Check sheet for the modelled part. Datum: model origin and axes. Units: mm. Face numbers are marked on the shaded views. A direction names the side the tool comes from. Round coordinates to 2 decimals unless told otherwise and drop trailing zeros. Write each loop counter-clockwise with the first axis right and the second up, starting at its lowest first coordinate (ties: lowest second). Pieces come first, ordered by that corner, then holes. Notation, with made-up numbers: (11, 66.25) -> (36, 66.25) arc R22 cw to (36, 99.25) -> close; hole circle Ø8 at (73, 68.5). An arc over 180 degrees is marked (long way). One line per item, written item: value. Start each with the question number.
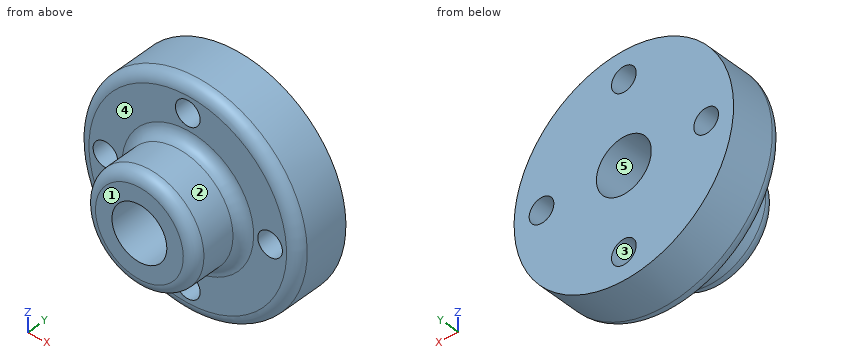
```python
from build123d import *

# Parameters (mm, degrees)
SKETCH1_R           = 254
BOSS_EXTRUDE1_DEPTH = 254
SKETCH2_R           = 508
BOSS_EXTRUDE2_DEPTH = 254
SKETCH3_R           = 127
CUT_EXTRUDE1_DEPTH  = 880.881810245
SKETCH4_R           = 57.15
CUT_EXTRUDE2_DEPTH  = 763
FILLET1_R           = 50.8


with BuildPart() as part:
    # Sketch1 → Boss-Extrude1 (new body)
    with BuildSketch(Plane(origin=(0, 0, 0), x_dir=(1, 0, 0), z_dir=(0, 1, 0))):
        with Locations(Location((0, 0, 0), (0, 0, 270))):
            Circle(SKETCH1_R)
    extrude(amount=BOSS_EXTRUDE1_DEPTH)

    # Sketch2 → Boss-Extrude2 (add)
    with BuildSketch(Plane(origin=(0, 254, 0), x_dir=(1, 0, 0), z_dir=(0, 1, 0))):
        with Locations(Location((0, 0, 0), (0, 0, 270))):
            Circle(SKETCH2_R)
    extrude(amount=BOSS_EXTRUDE2_DEPTH)

    # Sketch3 → Cut-Extrude1 (cut, through all)
    with BuildSketch(Plane.XZ):
        with Locations(Location((0, 0, 0), (0, 0, 270))):
            Circle(SKETCH3_R)
    extrude(amount=-CUT_EXTRUDE1_DEPTH, mode=Mode.SUBTRACT)

    # Sketch4 → Cut-Extrude2 (cut, through all)
    with BuildSketch(Plane.XZ.offset(-254)):
        with Locations(Location((0, -381, 0), (0, 0, 270))):
            Circle(SKETCH4_R)
        with Locations(Location((381, 0, 0), (0, 0, 270))):
            Circle(SKETCH4_R)
        with Locations(Location((0, 381, 0), (0, 0, 270))):
            Circle(SKETCH4_R)
        with Locations(Location((-381, 0, 0), (0, 0, 270))):
            Circle(SKETCH4_R)
    extrude(amount=-CUT_EXTRUDE2_DEPTH, mode=Mode.SUBTRACT)

    # Fillet1
    fillet1_edges = [part.edges().sort_by_distance(p)[0] for p in [
        (0, 0, -254),
        (0, 254, -254),
        (0, 254, -508),
    ]]
    fillet(fillet1_edges, radius=FILLET1_R)


solid = part.part
```
1. Access from +Z, -Z, +X, -X, +Y, -Y to the whole of each face (thin tool, end or side, straight path). Record for the marked faces 4 and 5.
2. Cross-section at C-C (y = 152). Record the cut outline in (x, z).
3. Material ranges on probe 1 along X at (y, z) = (437, 0); probe 2 along X at (y, z) = (140.5, 0); probe 3 along Y at (x, z) = (-377, -201), recorded low to high.
4. Cross-section at A-A (x = 0). Record the cut outline in (y, z).
5. Depth check by flat-ended pin: pin 1 Ø6 at (x, z) = (-163, 17) entering from -Y; pin 2 Ø3 at (y, z) = (218, -45.5) entering from +X; pin 3 Ø1.5 at (y, z) = (390.5, -88) entering from -X; pin 4 Ø3 at (x, z) = (-280, -150) entering from -Y. Enter the tip coordinate at first touch or a pass-through.
6. Cross-section at B-B (z = 0). Record the cut outline in (x, y).
7. Release check for a two-part mould opening along X. For the marked faces 1, 2 and 3 record: +X half, -X half, draft (parallel to the pull), parting line (faces both ways), or undercut.
Working result:
1. face 4: -Y
1. face 5: +Y, -Y
2. outline: circle Ø508 at (0, 0); hole circle Ø254 at (0, 0)
3. probe 1: x = -508 to -438.15, -323.85 to -127, 127 to 323.85, 438.15 to 508
3. probe 2: x = -254 to -127, 127 to 254
3. probe 3: y = 254 to 508
4. outline: (0, -203.2) arc R50.8 ccw to (50.8, -254) -> (203.2, -254) arc R50.8 cw to (254, -304.8) -> (254, -323.85) -> (508, -323.85) -> (508, -127) -> (0, -127) -> close; (0, 127) -> (508, 127) -> (508, 323.85) -> (254, 323.85) -> (254, 304.8) arc R50.8 cw to (203.2, 254) -> (50.8, 254) arc R50.8 ccw to (0, 203.2) -> close; (254, -457.2) arc R50.8 ccw to (304.8, -508) -> (508, -508) -> (508, -438.15) -> (254, -438.15) -> close; (254, 438.15) -> (508, 438.15) -> (508, 508) -> (304.8, 508) arc R50.8 ccw to (254, 457.2) -> close
5. pin 1: stops at y = 0
5. pin 2: stops at x = 252.69
5. pin 3: stops at x = -500.45
5. pin 4: stops at y = 254
6. outline: (-508, 304.8) arc R50.8 ccw to (-457.2, 254) -> (-438.15, 254) -> (-438.15, 508) -> (-508, 508) -> close; (-323.85, 254) -> (-304.8, 254) arc R50.8 cw to (-254, 203.2) -> (-254, 50.8) arc R50.8 ccw to (-203.2, 0) -> (-127, 0) -> (-127, 508) -> (-323.85, 508) -> close; (127, 0) -> (203.2, 0) arc R50.8 ccw to (254, 50.8) -> (254, 203.2) arc R50.8 cw to (304.8, 254) -> (323.85, 254) -> (323.85, 508) -> (127, 508) -> close; (438.15, 254) -> (457.2, 254) arc R50.8 ccw to (508, 304.8) -> (508, 508) -> (438.15, 508) -> close
7. face 1: draft
7. face 2: parting line
7. face 3: undercut
